Part model, mm, in its own coordinate system. A direction names the side the tool comes from. Round coordinates to 2 decimals unless told otherwise and drop trailing zeros. Write each loop counter-clockwise with the first axis right and the second up, starting at its lowest first coordinate (ties: lowest second). Pieces come first, ordered by that corner, then holes. Notation, with made-up numbers: M 15,73 L 54,73 A7 cw 54,79 Z; hole C 88.25,78.5 d6. An arc over 180 degrees is marked long. One line per question, with ' | ' between items. Start each with the question number.
1) Saw through at A-A (z = 114.3). List the corners of the cut face in (x, y), plus the area to 3 significant figures.
2) Drop flat-ended pins along their axis: pin 1 Ø15 at (x, y) = (-60.5, -31) entering from +Z; pin 2 Ø15 at (y, z) = (0, 114.3) entering from -X; pin 3 Ø2 at (y, z) = (29.5, 104) entering from -X; pin 4 Ø19 at (y, z) = (7, 114.5) entering from -X. Give the stop position or say it passes through.
3) Tool access for faces 4 (the face through (-19.05, -4, 102)), 5 (the face through (-50, -1, 25.4)), 6 (the face through (-70, 15.651, 13)): list every direction of +Z, -Z, +X, -X, +Y, -Y with a clear straight run to the whole face (end or side of a thin tool).
4) Saw through at D-D (x = -16). List the corners of the cut face in (y, z), plus the area to 3 significant figures.
5) Saw through at B-B (x = -60.5). List the corners of the cut face in (y, z).
6) Saw through at C-C (y = 0). List the corners of the cut face in (x, z).
7) Wall check: probe 1 along Z at (x, y) = (-9, 1); probe 2 along Z at (x, y) = (-20.5, 0); probe 3 along X at (y, z) = (-66, 112.5). Give the ranges that are in metal, low to high. Write a range as [from, to].
8) Mould opens along Y. For faces 1 (the face through (-76.2, 46, 13)), 2 (the face through (-22, 76.2, 60)), 3 (the face through (-70, -9.749, 13)) say: pulls with the +Y half, pulls with the -Y half, needs draft (parallel to the pull), parting line crosses it, or undercut.
```python
from build123d import *

# Parameters (mm, degrees)
F1_DEPTH = 76.2
F2_R     = 12.7
F3_DEPTH = 76.201
F5_DEPTH = 50.8
F6_R     = 19.05
F6_R_2   = 12.7
F7_DEPTH = 6.35


with BuildPart() as f1:
    # F0 (on Front) → F1 (new body, symmetric)
    with BuildSketch(Plane.XZ):
        Polygon((-25.4, 152.4), (-25.4, 25.4), (-76.2, 25.4), (-76.2, 0), (0, 0), (0, 152.4), align=None)
    extrude(amount=F1_DEPTH, both=True)

    # F2 (on face) → F3 (cut, through all)
    with BuildSketch(Plane.YZ):
        with Locations((0, 114.3)):
            Circle(F2_R)
    extrude(amount=-F3_DEPTH, mode=Mode.SUBTRACT)

    # F4 (on face) → F5 (cut)
    with BuildSketch(Plane.XY.offset(25.4)):
        with BuildLine():
            Line((-76.2, 15.650802), (-76.2, 2.950802))
            Line((-76.2, 2.950802), (-76.2, -9.749198))
            Line((-76.2, -9.749198), (-63.5, -9.749198))
            ThreePointArc((-63.5, -9.749198), (-50.8, 2.950802), (-63.5, 15.650802))
            Line((-63.5, 15.650802), (-76.2, 15.650802))
        make_face()
    extrude(amount=-F5_DEPTH, mode=Mode.SUBTRACT)

    # F6 (on face) → F7 (cut)
    with BuildSketch(Plane(origin=(-25.4, 0, 0), x_dir=(0, -1, 0), z_dir=(-1, 0, 0))):
        with Locations((0, 114.3)):
            Circle(F6_R)
        with Locations((0, 114.3)):
            Circle(F6_R_2, mode=Mode.SUBTRACT)
    extrude(amount=-F7_DEPTH, mode=Mode.SUBTRACT)


solid = f1.part
```
Answer key:
1) outline: M -25.4,-76.2 L 0,-76.2 L 0,-12.7 L -19.05,-12.7 L -19.05,-19.05 L -25.4,-19.05 Z; M -25.4,19.05 L -19.05,19.05 L -19.05,12.7 L 0,12.7 L 0,76.2 L -25.4,76.2 Z | area: 3,150 mm2
2) pin 1: stops at z = 25.4 | pin 2: passes through | pin 3: stops at x = -25.4 | pin 4: stops at x = -19.05
3) face 4: -X | face 5: +Z, -X, +Y, -Y | face 6: +Z, -Z, -X
4) outline: M -76.2,0 L 76.2,0 L 76.2,152.4 L -76.2,152.4 Z; hole C 0,114.3 d25.4 | area: 22,700 mm2
5) outline: M -76.2,0 L -9.39,0 L -9.39,25.4 L -76.2,25.4 Z; M 15.29,0 L 76.2,0 L 76.2,25.4 L 15.29,25.4 Z
6) outline: M -51.15,0 L 0,0 L 0,101.6 L -19.05,101.6 L -19.05,95.25 L -25.4,95.25 L -25.4,25.4 L -51.15,25.4 Z; M -25.4,133.35 L -19.05,133.35 L -19.05,127 L 0,127 L 0,152.4 L -25.4,152.4 Z
7) probe 1: z = [0, 101.64], [126.96, 152.4] | probe 2: z = [0, 95.25], [133.35, 152.4] | probe 3: x = [-25.4, 0]
8) face 1: needs draft | face 2: pulls with the +Y half | face 3: undercut
